Can you work these out from the model? Positions are in its coordinate system, mm. Face numbers are marked on the shaded views. A direction names the side the tool comes from. Round coordinates to 2 decimals unless told otherwise and drop trailing zeros. Order: outer loops, then holes, each group sorted by start corner. A loop starts at its lowest first (then second) coordinate and runs counter-clockwise, first axis right, second up.
Q1. If we section it at A-A (y = -5): Please give me the cut outline in (x, z), plus the area to 3 significant figures.
Q2. We'd pull the mould along X, two halves only. Please class the marked faces 3, 4 and 5: pulls with the +X half, pulls with the -X half, needs draft (parallel to the pull), parting line crosses it, or undercut.
Q3. If I drill on line 1 (Z direction, x = -25.75, y = -5); line 2 (Z direction, x = -25, y = -6.25); line 3 (Z direction, x = 3, y = -3.75), over which ranges is the centre line in solid material (lowest first)?
Q4. If we section it at B-B (z = -1): Please give me the cut outline in (x, y).
Q5. If we section it at D-D (x = -7.5): Please give me the cut outline in (y, z).
Q6. For the marked faces 1 and 2, which set-ups out of +Z, -Z, +X, -X, +Y, -Y let a thin tool reach every point of the face, with its end or its side?
Q7. If we section it at C-C (z = -12.5): Please give me the cut outline in (x, y).
Q8. Will these pins go through, and if not, where does the flat tip stop? P1, Ø10, axis at x = 10, z = -17, coming from the +Y side; P2, Ø3, axis at x = 0, y = -4.5, coming from the +Z side; P3, Ø4.5, axis at x = -19, z = -1, coming from the -Y side; P4, Ø3, axis at y = -5, z = -11, coming from the +X side.
from build123d import *

# Parameters (mm, degrees)
F0_R     = 2.75
F1_DEPTH = 10
F2_R     = 4
F3_DEPTH = 99
F4_R     = 2.5
F5_DEPTH = 25
F6_R     = 2.5
F7_DEPTH = 25


with BuildPart() as f1:
    # F0 (on Front) → F1 (new body)
    with BuildSketch(Plane.XZ):
        Polygon((-19, 24), (-39, 24), (-39, -26), (39, -26), (39, 24), (19, 24), (19, 4), (-19, 4), align=None)
        with Locations((-19, -21)):
            Circle(F0_R, mode=Mode.SUBTRACT)
        with Locations((19, -21)):
            Circle(F0_R, mode=Mode.SUBTRACT)
        with Locations((-19, -1)):
            Circle(F0_R, mode=Mode.SUBTRACT)
        with Locations((19, -1)):
            Circle(F0_R, mode=Mode.SUBTRACT)
    extrude(amount=F1_DEPTH)

    # F2 (on face) → F3 (cut)
    with BuildSketch(Plane(origin=(-39, 0, 0), x_dir=(0, -1, 0), z_dir=(-1, 0, 0))):
        with Locations((5, 18.786615)):
            Circle(F2_R)
    extrude(amount=-F3_DEPTH, mode=Mode.SUBTRACT)

    # F4 (on face) → F5 (cut)
    with BuildSketch(Plane(origin=(-39, 0, 0), x_dir=(0, -1, 0), z_dir=(-1, 0, 0))):
        with Locations((5, -11)):
            Circle(F4_R)
    extrude(amount=-F5_DEPTH, mode=Mode.SUBTRACT)

    # F6 (on face) → F7 (cut)
    with BuildSketch(Plane.YZ.offset(39)):
        with Locations((-5, -11)):
            Circle(F6_R)
    extrude(amount=-F7_DEPTH, mode=Mode.SUBTRACT)


solid = f1.part
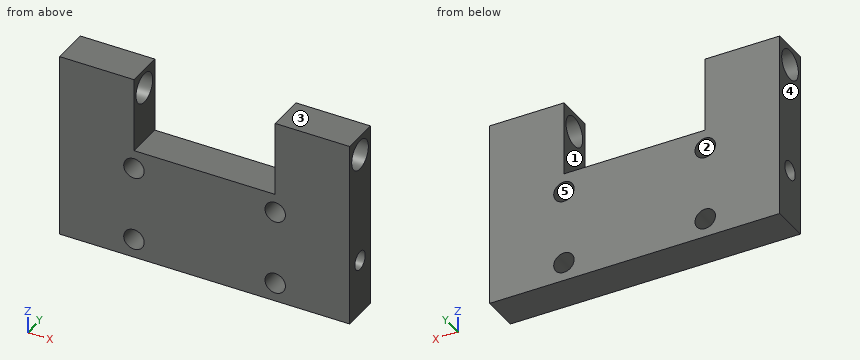
Solution:
1. outline: (-39, -26) - (39, -26) - (39, -13.5) - (14, -13.5) - (14, -8.5) - (39, -8.5) - (39, 14.79) - (19, 14.79) - (19, 4) - (-19, 4) - (-19, 14.79) - (-39, 14.79) - (-39, -8.5) - (-14, -8.5) - (-14, -13.5) - (-39, -13.5) - close; (-39, 22.79) - (-19, 22.79) - (-19, 24) - (-39, 24) - close; (19, 22.79) - (39, 22.79) - (39, 24) - (19, 24) - close; hole circle Ø5.5 at (-19, -21); hole circle Ø5.5 at (-19, -1); hole circle Ø5.5 at (19, -21); hole circle Ø5.5 at (19, -1)
1. area: 2,470 mm2
2. face 3: needs draft
2. face 4: pulls with the -X half
2. face 5: undercut
3. line 1: z = -26 to -13.5, -8.5 to 14.79, 22.79 to 24
3. line 2: z = -26 to -13.17, -8.83 to 14.99, 22.59 to 24
3. line 3: z = -26 to 4
4. outline: (-39, -10) - (-21.75, -10) - (-21.75, 0) - (-39, 0) - close; (-16.25, -10) - (16.25, -10) - (16.25, 0) - (-16.25, 0) - close; (21.75, -10) - (39, -10) - (39, 0) - (21.75, 0) - close
5. outline: (-10, -26) - (0, -26) - (0, 4) - (-10, 4) - close
6. face 1: +Z, +Y, -Y
6. face 2: +Y, -Y
7. outline: (-39, -10) - (39, -10) - (39, -7) - (14, -7) - (14, -3) - (39, -3) - (39, 0) - (-39, 0) - (-39, -3) - (-14, -3) - (-14, -7) - (-39, -7) - close
8. P1: stops at y = 0
8. P2: stops at z = 4
8. P3: passes through
8. P4: stops at x = 14
